from build123d import *

# Parameters (mm, degrees)
SKETCH1_R            = 150
BOSS_EXTRUDE1_DEPTH  = 6.35
M6_CLEARANCE_HOLE1_D = 6.4
CIRPATTERN1_COUNT    = 8


with BuildPart() as part:
    # Sketch1 → Boss-Extrude1 (new body)
    with BuildSketch(Plane(origin=(0, 0, 0), x_dir=(1, 0, 0), z_dir=(0, 1, 0))):
        with Locations(Location((0, 0, 0), (0, 0, 270))):
            Circle(SKETCH1_R)
    extrude(amount=-BOSS_EXTRUDE1_DEPTH)

    # M6 Clearance Hole1 (through all)
    with Locations(Plane(origin=(-30, 0, -130), x_dir=(0, 0, 1), z_dir=(0, 1, 0))):
        with Locations((0, 0), (0, 60)):
            m6_clearance_hole1 = Hole(M6_CLEARANCE_HOLE1_D / 2)

    # CirPattern1: M6 Clearance Hole1 ×8 about axis
    cirpattern1_axis = Axis((0, 0, 0), (0, 1, 0))
    for i in range(1, CIRPATTERN1_COUNT):
        add(m6_clearance_hole1.rotate(cirpattern1_axis, i * 360 / CIRPATTERN1_COUNT), mode=Mode.SUBTRACT)


solid = part.part
The model under review builds one solid part; all positions refer to its coordinate system, in mm. Round coordinates to 2 decimals unless told otherwise and drop trailing zeros. Loops run counter-clockwise (first coordinate to the right, second up) from the corner with the lowest first, then second, coordinate; pieces in that order, holes last. Notation, with made-up numbers: (57, 82) -> (86, 82) arc R21 cw to (86, 117) -> close; hole circle Ø4 at (81.25, 47.25). An arc over 180 degrees is marked (long way). Write item = value, one per line. Start each with the question number.
Item 1: Take a section at B-B on x = -39.5. Give the boundary of the cut face in (y, z).
Item 2: Take a section at C-C on z = -46.5. Give the boundary of the cut face in (x, y).
Item 3: Insertion check: pin 1 (3 mm diameter, centred on y = -0.5, z = 29.5, fed in from +X). The pin has a flat end and moves straight along its axis. Give the tip position at first contact, or say it passes through.
Item 4: Mouldability with a two-part tool opening along Z and no side actions: class faces 1 (the cylindrical face through (109.965, -3.219, -70.292)), 2 (the flat face through (2, 0, -2)) as released by +Z, released by -Z, zero draft, split by the parting line, or undercut.
Item 5: Take a section at A-A on y = -2.5. Count the separate pieces of the cut face and the enclosed holes in it, plus the area to 3 significant figures.
Item 6: To check wall thickness, follow L1, parallel to Z at x = -68, y = -1.75; L2, parallel to Z at x = 130, y = -5; L3, parallel to X at y = -2.5, z = 114.5. State the ranges of each line that lie inside material, in increasing order.
Result:
q1.outline = (-6.35, -144.71) -> (0, -144.71) -> (0, 144.71) -> (-6.35, 144.71) -> close
q2.outline = (-142.61, -6.35) -> (142.61, -6.35) -> (142.61, 0) -> (-142.61, 0) -> close
q3.pin_1 = 147.36
q4.face_1 = undercut
q4.face_2 = zero draft
q5.separate_pieces = 1
q5.enclosed_holes = 16
q5.area = 70,200 mm²
q6.L1 = -133.7 to -114.84, -111.44 to 111.44, 114.84 to 133.7
q6.L2 = -74.83 to -33.2, -26.8 to 26.8, 33.2 to 74.83
q6.L3 = -96.9 to -73.61, -67.82 to 67.82, 73.61 to 96.9
